Geometry check sheet. Reference: the model listing, model coordinates, mm. A direction names the side the tool comes from. Coordinates: 2 decimals unless noted, no trailing zeros. Write each loop counter-clockwise with the first axis right and the second up, starting at its lowest first coordinate (ties: lowest second). Pieces come first, ordered by that corner, then holes. Notation, with made-up numbers: (17.5, -27.5) -> (59.5, -27.5) arc R12 ccw to (59.5, -14.5) -> close; hole circle Ø9 at (22.5, -13.75). An arc over 180 degrees is marked (long way). Answer in a Markdown table with one row per item. Add a question column.
1. Cross-section at C-C on z = -2.25. Record the cut outline in (x, y).
2. Depth check by flat-ended pin: P1, Ø6.5, axis at x = 0, y = 0, coming from the -Z side; P2, Ø5, axis at y = 3, z = -0.5, coming from the -X side; P3, Ø2, axis at x = -13, y = -11, coming from the +Z side; P4, Ø2, axis at y = 4.5, z = 2.5, coming from the +X side. Enter the tip coordinate at first touch or a pass-through.
3. Mould release check, pull along Y, two halves, no side actions. Record for faces 4 (the cylindrical face through (-4.336, -19.524, -1.972)), 5 (the flat face through (9, -4, 0)), 6 (the cylindrical face through (-2.17, 9.76, -4.52)): pulls with the +Y half, pulls with the -Y half, needs draft (parallel to the pull), parting line crosses it, or undercut.
4. Cross-section at D-D on y = -15.5. Record the cut outline in (x, z), and give its area (3 significant figures).
5. Set-up check for faces 1 (the flat face through (4, -2, 3.5)), 2 (the cylindrical face through (-1.172, 8.923, 1.726)), 3 (the flat face through (0, 18, -4)): record each of +Z, -Z, +X, -X, +Y, -Y from which the full face is reachable in a straight line by a thin tool's end or side.
6. Scan lines: L1, parallel to Y at x = 0, z = -1; L2, parallel to X at y = 0, z = -3.8; L3, parallel to Z at x = -15, y = -6. Record each from-to range of solid material in increasing order. Write a range as from..to.
7. Cross-section at A-A on y = 0. Record the cut outline in (x, z).
```python
from build123d import *

# Parameters (mm, degrees)
F0_R     = 9
F0_R_2   = 4
F1_DEPTH = 3.5
F0_R_3   = 20
F2_DEPTH = 6
F3_R     = 10
F3_R_2   = 4
F4_DEPTH = 3
F3_R_3   = 20
F3_R_4   = 17.5
F5_DEPTH = 2


with BuildPart() as f1:
    # F0 (on Top) → F1 (new body)
    with BuildSketch(Plane.XY):
        Circle(F0_R)
        Circle(F0_R_2, mode=Mode.SUBTRACT)
    extrude(amount=F1_DEPTH)

    # F0 (on Top) → F2 (join)
    with BuildSketch(Plane.XY):
        Circle(F0_R_3)
        Circle(F0_R, mode=Mode.SUBTRACT)
        Circle(F0_R)
        Circle(F0_R_2, mode=Mode.SUBTRACT)
    extrude(amount=-F2_DEPTH)

    # F3 (on face) → F4 (cut)
    with BuildSketch(Plane(origin=(0, 0, -6), x_dir=(1, 0, 0), z_dir=(0, 0, -1))):
        Circle(F3_R)
        Circle(F3_R_2, mode=Mode.SUBTRACT)
    extrude(amount=-F4_DEPTH, mode=Mode.SUBTRACT)

    # F3 (on face) → F5 (cut)
    with BuildSketch(Plane(origin=(0, 0, -6), x_dir=(1, 0, 0), z_dir=(0, 0, -1))):
        Circle(F3_R_3)
        Circle(F3_R_4, mode=Mode.SUBTRACT)
    extrude(amount=-F5_DEPTH, mode=Mode.SUBTRACT)


solid = f1.part
```
Results found:
| question | item | result |
|---|---|---|
| 1 | outline | circle Ø40 at (0, 0); hole circle Ø8 at (0, 0) |
| 2 | P1 | passes through |
| 2 | P2 | stops at x = -19.99 |
| 2 | P3 | stops at z = 0 |
| 2 | P4 | stops at x = 8.29 |
| 3 | face 4 | parting line crosses it |
| 3 | face 5 | needs draft |
| 3 | face 6 | undercut |
| 4 | outline | (-12.64, -4) -> (-8.12, -4) -> (-8.12, -6) -> (8.12, -6) -> (8.12, -4) -> (12.64, -4) -> (12.64, 0) -> (-12.64, 0) -> close |
| 4 | area | 134 mm^2 |
| 5 | face 1 | +Z, +X, -X, +Y, -Y |
| 5 | face 2 | +Z |
| 5 | face 3 | -Z |
| 6 | L1 | y = -20..-4, 4..20 |
| 6 | L2 | x = -20..-10, 10..20 |
| 6 | L3 | z = -6..0 |
| 7 | outline | (-20, -4) -> (-17.5, -4) -> (-17.5, -6) -> (-10, -6) -> (-10, -3) -> (-4, -3) -> (-4, 3.5) -> (-9, 3.5) -> (-9, 0) -> (-20, 0) -> close; (4, -3) -> (10, -3) -> (10, -6) -> (17.5, -6) -> (17.5, -4) -> (20, -4) -> (20, 0) -> (9, 0) -> (9, 3.5) -> (4, 3.5) -> close |
